from build123d import *

# Parameters (mm, degrees)
SKETCH_W          = 46
SKETCH_H          = 48
SKETCH_R          = 1.6
SKETCH_R_2        = 6.1
PAD_DEPTH         = 5
SKETCH001_W       = 46
SKETCH001_H       = 6
PAD001_DEPTH      = 60
PAD001_DEPTH_BACK = 5
SKETCH002_W       = 17.3
SKETCH002_H       = 65
PAD002_DEPTH      = 18
POCKET_DEPTH      = 8
SKETCH004_R       = 2.6
POCKET001_DEPTH   = 72.001
PAD003_DEPTH      = 3
PAD004_DEPTH      = 3
SKETCH007_W       = 7.25
SKETCH007_H       = 6
SKETCH007_R       = 1.6
PAD005_DEPTH      = 3


with BuildPart() as part:
    # Sketch → Pad (new body)
    with BuildSketch(Plane.XY):
        with Locations((0, -2)):
            Rectangle(SKETCH_W, SKETCH_H)
        with Locations((-7.75, 13.423394)):
            Circle(SKETCH_R, mode=Mode.SUBTRACT)
        with Locations((7.75, 13.423394)):
            Circle(SKETCH_R, mode=Mode.SUBTRACT)
        with Locations((-15.5, 0)):
            Circle(SKETCH_R, mode=Mode.SUBTRACT)
        with Locations((-7.75, -13.423394)):
            Circle(SKETCH_R, mode=Mode.SUBTRACT)
        with Locations((7.75, -13.423394)):
            Circle(SKETCH_R, mode=Mode.SUBTRACT)
        with Locations((15.5, 0)):
            Circle(SKETCH_R, mode=Mode.SUBTRACT)
        with Locations((0, -7)):
            Circle(SKETCH_R_2, mode=Mode.SUBTRACT)
    extrude(amount=PAD_DEPTH)

    # Sketch001 → Pad001 (new body, two sides)
    with BuildSketch(Plane.XY.offset(5)) as pad001_sk:
        with Locations((0, -29)):
            Rectangle(SKETCH001_W, SKETCH001_H)
    extrude(amount=PAD001_DEPTH)
    extrude(pad001_sk.sketch, amount=-PAD001_DEPTH_BACK)

    # Sketch002 → Pad002 (new body)
    with BuildSketch(Plane.XZ.offset(32)):
        with Locations((0, 32.5)):
            Rectangle(SKETCH002_W, SKETCH002_H)
    extrude(amount=PAD002_DEPTH)

    # Sketch003 → Pocket (cut)
    with BuildSketch(Plane(origin=(0, -26, 0), x_dir=(-1, 0, 0), z_dir=(0, 1, 0))):
        Polygon((4.5, 50), (2.25, 53.897114), (-2.25, 53.897114), (-4.5, 50), (-2.25, 46.102886), (2.25, 46.102886), align=None)
        Polygon((4.5, 20), (2.25, 23.897114), (-2.25, 23.897114), (-4.5, 20), (-2.25, 16.102886), (2.25, 16.102886), align=None)
    extrude(amount=-POCKET_DEPTH, mode=Mode.SUBTRACT)

    # Sketch004 → Pocket001 (cut, through all)
    with BuildSketch(Plane.XZ.offset(50)):
        with Locations((0, 50)):
            Circle(SKETCH004_R)
        with Locations((0, 20)):
            Circle(SKETCH004_R)
    extrude(amount=-POCKET001_DEPTH, mode=Mode.SUBTRACT)

    # Sketch005 → Pad003 (new body)
    with BuildSketch(Plane(origin=(-23, 0, 0), x_dir=(0, -1, 0), z_dir=(-1, 0, 0))):
        Polygon((-22, 5), (26, 5), (26, 53), align=None)
    extrude(amount=-PAD003_DEPTH)

    # Sketch006 → Pad004 (new body)
    with BuildSketch(Plane.YZ.offset(23)):
        Polygon((22, 5), (-26, 5), (-26, 53), align=None)
    extrude(amount=-PAD004_DEPTH)

    # Sketch007 → Pad005 (new body)
    with BuildSketch(Plane(origin=(0, 0, 0), x_dir=(1, 0, 0), z_dir=(0, 0, -1))):
        with Locations((-26.625, 18)):
            Rectangle(SKETCH007_W, SKETCH007_H)
        with Locations((-27.25, 18)):
            Circle(SKETCH007_R, mode=Mode.SUBTRACT)
        with Locations((26.625, -18)):
            Rectangle(SKETCH007_W, SKETCH007_H)
        with Locations((27.25, -18)):
            Circle(SKETCH007_R, mode=Mode.SUBTRACT)
    extrude(amount=-PAD005_DEPTH)


solid = part.part
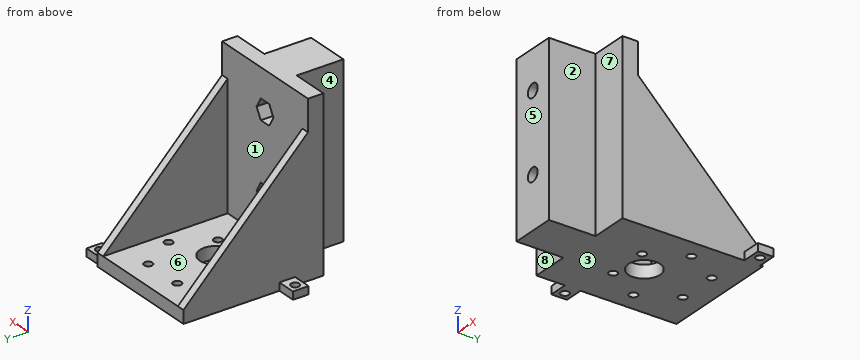
Could you check a few things on this model? Use its own coordinates, in mm. Face numbers are marked on the shaded views. A direction names the side the tool comes from. Coordinates: 2 decimals unless noted, no trailing zeros. Loops run counter-clockwise (first coordinate to the right, second up) from the corner with the lowest first, then second, coordinate; pieces in that order, holes last.
1. Imagine slicing it at D-D (x = -27.25). Please give me the cut outline in (y, z).
2. I need wall thicknesses on L1, parallel to Z at x = 0, y = -42; L2, parallel to Y at x = -7, z = 3; L3, parallel to X at y = 18, z = 1. Which ranges of each line are inside material? Lowest first, please.
3. For the marked faces 5, 6, 7 and 8, which set-ups out of +Z, -Z, +X, -X, +Y, -Y let a thin tool reach every point of the face, with its end or its side?
4. Imagine slicing it at B-B (x = 15.5). Please give me the cut outline in (y, z).
5. We'd pull the mould along X, two halves only. Please class the marked faces 1, 2, 3 and 4: released by +X, released by -X, zero draft, split by the parting line, or undercut.
6. Imagine slicing it at C-C (z = 13). Please give me the cut outline in (x, y).
7. For P1, Ø12, axis at x = -23, z = 13, coming from the +Y side; P2, Ø6.5, axis at x = -27.5, y = -19, coming from the +Z side; P3, Ø4, axis at x = 12, z = 25.5, coming from the +Y side; P4, Ø4, axis at x = 0, z = 20, coming from the +Y side, each with a flat end and sliding along its axis, tell me the tip position at first contact or that it passes through.
8. Imagine slicing it at A-A (y = 18). Please give me the cut outline in (x, z).
Computed values:
1. outline: (-21, 0) - (-19.6, 0) - (-19.6, 3) - (-21, 3) - close; (-16.4, 0) - (-15, 0) - (-15, 3) - (-16.4, 3) - close
2. L1: z = 0 to 17.4, 22.6 to 47.4, 52.6 to 65
2. L2: y = -50 to -14.84, -12.01 to 12.01, 14.84 to 22
2. L3: x = -23 to 25.65, 28.85 to 30.25
3. face 5: +Z, -Z, +X, -X, -Y
3. face 6: +Z, +Y
3. face 7: +Z, -Z, +X, -Y
3. face 8: +Z, -Z, -X, -Y
4. outline: (-32, 0) - (-1.6, 0) - (-1.6, 5) - (-26, 5) - (-26, 65) - (-32, 65) - close; (1.6, 0) - (22, 0) - (22, 5) - (1.6, 5) - close
5. face 1: undercut
5. face 2: released by +X
5. face 3: zero draft
5. face 4: released by -X
6. outline: (-23, -32) - (-8.65, -32) - (-8.65, -50) - (8.65, -50) - (8.65, -32) - (23, -32) - (23, 14) - (20, 14) - (20, -26) - (-20, -26) - (-20, 14) - (-23, 14) - close
7. P1: stops at y = 20
7. P2: stops at z = 3
7. P3: stops at y = -26
7. P4: passes through
8. outline: (-23, 0) - (25.65, 0) - (25.65, 3) - (23, 3) - (23, 9) - (20, 9) - (20, 5) - (-20, 5) - (-20, 9) - (-23, 9) - close; (28.85, 0) - (30.25, 0) - (30.25, 3) - (28.85, 3) - close
